Part model, mm, in its own coordinate system. Face numbers are marked on the shaded views. A direction names the side the tool comes from. Coordinates: 2 decimals unless noted, no trailing zeros. Order: outer loops, then holes, each group sorted by start corner. A loop starts at its lowest first (then second) coordinate and runs counter-clockwise, first axis right, second up.
1) Cut at C-C (x = 3). List the corners of the cut face in (y, z).
2) Cut at D-D (x = 35.5). List the corners of the cut face in (y, z).
3) Tool access for the marked faces 4 and 5: list every direction of +Z, -Z, +X, -X, +Y, -Y with a clear straight run to the whole face (end or side of a thin tool).
4) Pin check, flat tips, straight feed: pin 1 Ø10 at (x, y) = (6, -2.5) entering from -Z; pin 2 Ø10 at (y, z) = (43.5, -45.5) entering from +X; pin 3 Ø12 at (y, z) = (12.5, 0.5) entering from -X; pin 4 Ø6 at (y, z) = (-36, -33) entering from -X. Stop position of each tip, or through.
5) Wall check: L1, parallel to Y at x = 9.25, z = 0; L2, parallel to X at y = 40.5, z = -13; L3, parallel to Y at x = 9, z = -22. Give the ranges that are in metal, low to high.
6) Mould opens along Y. For the marked faces 1, 2 and 3 say: +Y half, -Y half, draft (parallel to the pull), parting line (faces both ways), or undercut.
```python
from build123d import *

# Parameters (mm, degrees)
SKETCH_1_R      = 50
SKETCH_1_R_2    = 45
EXTRUDE_1_DEPTH = 30
SKETCH_2_R      = 60
EXTRUDE_2_DEPTH = 10
CHAMFER_1_SIZE  = 10


with BuildPart() as part:
    # Эскиз1 → Бобышка-Вытянуть1 (new body)
    with BuildSketch(Plane(origin=(0, 0, 0), x_dir=(0, 0, -1), z_dir=(1, 0, 0))):
        Circle(SKETCH_1_R)
        Circle(SKETCH_1_R_2, mode=Mode.SUBTRACT)
    extrude(amount=EXTRUDE_1_DEPTH)

    # Эскиз2 → Бобышка-Вытянуть2 (add)
    with BuildSketch(Plane(origin=(30, 0, 0), x_dir=(0, 0, -1), z_dir=(1, 0, 0))):
        Circle(SKETCH_2_R)
    extrude(amount=EXTRUDE_2_DEPTH)

    # Фаска1
    chamfer_1_edges = [part.edges().sort_by_distance(p)[0] for p in [
        (40, 0, 60),
    ]]
    chamfer(chamfer_1_edges, length=CHAMFER_1_SIZE - 0.0001)  # a hair under: the kernel refuses the full size


solid = part.part
```
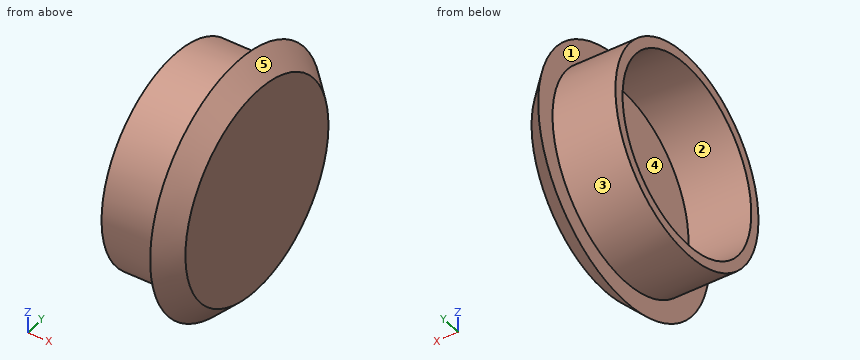
Geometry check:
1. outline: circle Ø100 at (0, 0); hole circle Ø90 at (0, 0)
2. outline: circle Ø109 at (0, 0)
3. face 4: -X
3. face 5: +X
4. pin 1: stops at z = -50
4. pin 2: stops at x = 32.05
4. pin 3: stops at x = 30
4. pin 4: stops at x = 0
5. L1: y = -50 to -45, 45 to 50
5. L2: x = 30 to 40
5. L3: y = -44.9 to -39.26, 39.26 to 44.9
6. face 1: draft
6. face 2: undercut
6. face 3: parting line
